from build123d import *

# Parameters (mm, degrees)
ESQUISSE1_W             = 23
ESQUISSE1_H             = 15.2
ESQUISSE1_R             = 1.5
BOSS_EXTRU_1_DEPTH      = 3
ESQUISSE2_W             = 23
ESQUISSE2_H             = 5
BOSS_EXTRU_2_DEPTH      = 10
ESQUISSE4_W             = 3
ESQUISSE4_H             = 31.2
BOSS_EXTRU_3_DEPTH      = 35
CONG_1_R                = 10
ESQUISSE7_W             = 10.405823793
ESQUISSE7_H             = 15
BOSS_EXTRU_4_DEPTH      = 3
ESQUISSE8_W             = 4
ESQUISSE8_H             = 15
BOSS_EXTRU_5_DEPTH      = 9.7
ESQUISSE9_W             = 26.005823793
ESQUISSE9_H             = 15
BOSS_EXTRU_6_DEPTH      = 5.52
ESQUISSE10_R            = 1.5
ENL_V_MAT_EXTRU_2_DEPTH = 5.52
ESQUISSE5_R             = 1.5
ENL_V_MAT_EXTRU_3_DEPTH = 10


with BuildPart() as part:
    # Esquisse1 → Boss.-Extru.1 (new body)
    with BuildSketch(Plane(origin=(0, 0, 0), x_dir=(0, 0, -1), z_dir=(1, 0, 0))):
        with Locations((11.5, -7.6)):
            Rectangle(ESQUISSE1_W, ESQUISSE1_H)
        with Locations((6.5, -5)):
            Circle(ESQUISSE1_R, mode=Mode.SUBTRACT)
        with Locations(Location((16.5, -5, 0), (0, 0, 180))):
            Circle(ESQUISSE1_R, mode=Mode.SUBTRACT)
    extrude(amount=BOSS_EXTRU_1_DEPTH)

    # Esquisse2 → Boss.-Extru.2 (add)
    with BuildSketch(Plane.ZY):
        with Locations((-11.5, -12.7)):
            Rectangle(ESQUISSE2_W, ESQUISSE2_H)
    boss_extru_2 = extrude(amount=BOSS_EXTRU_2_DEPTH)

    # Esquisse4 → Boss.-Extru.3 (add)
    with BuildSketch(Plane.XZ.offset(15.2)):
        with Locations((-8.5, -11.5)):
            Rectangle(ESQUISSE4_W, ESQUISSE4_H)
    boss_extru_3 = extrude(amount=BOSS_EXTRU_3_DEPTH)

    # Congé1
    cong_1_edges = [part.edges().sort_by_distance(p)[0] for p in [
        (-8.5, -50.2, -27.1),
        (-8.5, -50.2, 4.1),
    ]]
    fillet(cong_1_edges, radius=CONG_1_R)

    # Esquisse7 → Boss.-Extru.4 (add, through all)
    with BuildSketch(Plane(origin=(-7, 0, 0), x_dir=(0, 0, -1), z_dir=(1, 0, 0))):
        with Locations((-9.302911897, -27.2)):
            Rectangle(ESQUISSE7_W, ESQUISSE7_H)
    boss_extru_4 = extrude(amount=-BOSS_EXTRU_4_DEPTH)

    # Esquisse8 → Boss.-Extru.5 (add)
    with BuildSketch(Plane(origin=(-7, 0, 0), x_dir=(0, 0, -1), z_dir=(1, 0, 0))):
        with Locations((-12.505823793, -27.2)):
            Rectangle(ESQUISSE8_W, ESQUISSE8_H)
    boss_extru_5 = extrude(amount=BOSS_EXTRU_5_DEPTH)

    # Esquisse9 → Boss.-Extru.6 (add)
    with BuildSketch(Plane(origin=(2.7, 0, 0), x_dir=(0, 0, -1), z_dir=(1, 0, 0))):
        with Locations((-1.502911897, -27.2)):
            Rectangle(ESQUISSE9_W, ESQUISSE9_H)
    boss_extru_6 = extrude(amount=BOSS_EXTRU_6_DEPTH)

    # Symétrie1: Boss.-Extru.2, Boss.-Extru.3, Boss.-Extru.4, Boss.-Extru.5, Boss.-Extru.6 across plane
    add(boss_extru_2.mirror(Plane(origin=(8.22, -19.7, -11.5), x_dir=(1, 0, 0), z_dir=(0, 0, 1))))
    add(boss_extru_3.mirror(Plane(origin=(8.22, -19.7, -11.5), x_dir=(1, 0, 0), z_dir=(0, 0, 1))))
    add(boss_extru_4.mirror(Plane(origin=(8.22, -19.7, -11.5), x_dir=(1, 0, 0), z_dir=(0, 0, 1))))
    add(boss_extru_5.mirror(Plane(origin=(8.22, -19.7, -11.5), x_dir=(1, 0, 0), z_dir=(0, 0, 1))))
    add(boss_extru_6.mirror(Plane(origin=(8.22, -19.7, -11.5), x_dir=(1, 0, 0), z_dir=(0, 0, 1))))

    # Esquisse10 → Enlèv. mat.-Extru.2 (cut)
    with BuildSketch(Plane(origin=(8.22, 0, 0), x_dir=(0, 0, -1), z_dir=(1, 0, 0))):
        with BuildLine():
            ThreePointArc((3, -27.2), (1.5, -25.7), (0, -27.2))
            Line((0, -27.2), (3, -27.2))
        make_face()
        with BuildLine():
            Line((3, -27.2), (0, -27.2))
            ThreePointArc((0, -27.2), (1.5, -28.7), (3, -27.2))
        make_face()
        with BuildLine():
            Line((-4.4, -21.3), (-4.4, -27.2))
            Line((-4.4, -27.2), (0, -27.2))
            ThreePointArc((0, -27.2), (1.5, -25.7), (3, -27.2))
            Line((3, -27.2), (18.3, -27.2))
            Line((18.3, -27.2), (18.3, -21.3))
            Line((18.3, -21.3), (-4.4, -21.3))
        make_face()
        with BuildLine():
            Line((0, -27.2), (-4.4, -27.2))
            Line((-4.4, -27.2), (-4.4, -33.1))
            Line((-4.4, -33.1), (18.3, -33.1))
            Line((18.3, -33.1), (18.3, -27.2))
            Line((18.3, -27.2), (3, -27.2))
            ThreePointArc((3, -27.2), (1.5, -28.7), (0, -27.2))
        make_face()
        with Locations((-7.4, -27.2)):
            Circle(ESQUISSE10_R)
        with Locations((21.3, -27.2)):
            Circle(ESQUISSE10_R)
    extrude(amount=-ENL_V_MAT_EXTRU_2_DEPTH, mode=Mode.SUBTRACT)

    # Esquisse5 → Enlèv. mat.-Extru.3 (cut)
    with BuildSketch(Plane(origin=(-7, 0, 0), x_dir=(0, 0, -1), z_dir=(1, 0, 0))):
        with Locations((6.5, -45.2)):
            Circle(ESQUISSE5_R)
        with Locations((1.5, -27.2)):
            Circle(ESQUISSE5_R)
        with Locations((16.5, -45.2)):
            Circle(ESQUISSE5_R)
        with Locations((21.5, -27.2)):
            Circle(ESQUISSE5_R)
    extrude(amount=-ENL_V_MAT_EXTRU_3_DEPTH, mode=Mode.SUBTRACT)


solid = part.part
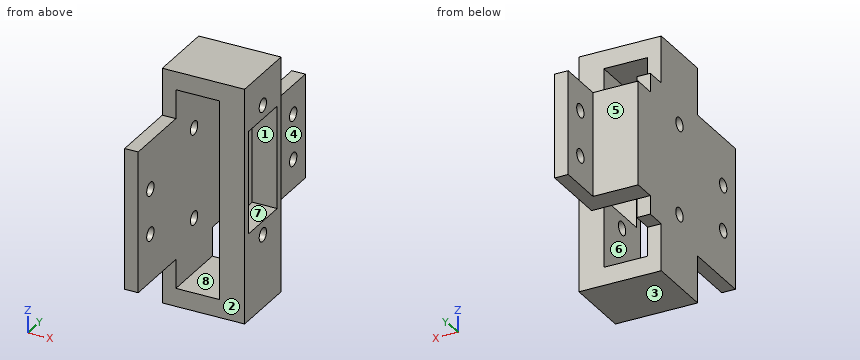
Read the model definition and answer for the solid it produces. Units are mm, in the model's axes. Face numbers are marked on the shaded views. A direction names the side the tool comes from. Round coordinates to 2 decimals unless told otherwise and drop trailing zeros. Order: outer loops, then holes, each group sorted by start corner. A loop starts at its lowest first (then second) coordinate and runs counter-clockwise, first axis right, second up.
1) The part is cut by section C-C on z = -1.5. Write down the section's boundary in (x, y).
2) The part is cut by section B-B on x = 1. Write down the section's boundary in (y, z).
3) For the marked faces 4, 5, 6, 7 and 8, determine the directions among +Z, -Z, +X, -X, +Y, -Y from which every point of the face is accessible in a straight line to the end or side of a thin tool.
4) The part is cut by section D-D on y = -5. Write down the section's boundary in (x, z), plus the area to 3 significant figures.
5) Flat-ended cylindrical pins translate along their axes: pin 1 (0.9 mm diameter, centred on x = -9, y = -43, fed in from -Z); pin 2 (8 mm diameter, centred on y = -4, z = -7, fed in from -X); pin 3 (4 mm diameter, centred on x = -4, z = -1.5, fed in from -Y). Find the tip coordinate at first contact, or state that the pin passes through.
6) The part is cut by section A-A on z = 7.4. Write down the section's boundary in (x, y), plus the area to 3 significant figures.
7) The mould has two halves that part along Z. Classify the marked faces 1, 2 and 3: released by +Z, released by -Z, zero draft, split by the parting line, or undercut.
8) Straight lines are drawn through the part: L1, parallel to Y at x = -8.2, z = -6.5; L2, parallel to Y at x = 7.1, z = 7.4; L3, parallel to Z at x = -0.75, y = -22. For each, find the intervals that lie inside material, in ascending order.
Resolved:
1. outline: (-10, -50.2) - (-7, -50.2) - (-7, -28.7) - (-10, -28.7) - close; (-10, -25.7) - (-7, -25.7) - (-7, -15.2) - (3, -15.2) - (3, 0) - (0, 0) - (0, -10.2) - (-10, -10.2) - close; (2.7, -34.7) - (8.22, -34.7) - (8.22, -33.1) - (2.7, -33.1) - close; (2.7, -21.3) - (8.22, -21.3) - (8.22, -19.7) - (2.7, -19.7) - close
2. outline: (-34.7, -37.51) - (-19.7, -37.51) - (-19.7, -33.51) - (-34.7, -33.51) - close; (-34.7, 10.51) - (-19.7, 10.51) - (-19.7, 14.51) - (-34.7, 14.51) - close; (-15.2, -23) - (0, -23) - (0, 0) - (-15.2, 0) - close; hole circle Ø3 at (-5, -16.5); hole circle Ø3 at (-5, -6.5)
3. face 4: +Z, -Z, +X, +Y
3. face 5: +Z, -Z, -X, +Y
3. face 6: -Y
3. face 7: +X
3. face 8: +Y, -Y
4. outline: (0, -23) - (3, -23) - (3, -18) - (0, -18) - close; (0, -15) - (3, -15) - (3, -8) - (0, -8) - close; (0, -5) - (3, -5) - (3, 0) - (0, 0) - close
4. area: 51.0 mm2
5. pin 1: stops at z = -27.1
5. pin 2: stops at x = 0
5. pin 3: stops at y = -15.2
6. outline: (-10, -34.7) - (-7, -34.7) - (-7, -19.7) - (-10, -19.7) - close; (2.7, -34.7) - (8.22, -34.7) - (8.22, -28.7) - (2.7, -28.7) - close; (2.7, -25.7) - (8.22, -25.7) - (8.22, -19.7) - (2.7, -19.7) - close
6. area: 111 mm2
7. face 1: undercut
7. face 2: zero draft
7. face 3: released by -Z
8. L1: y = -50.2 to -46.7, -43.7 to -10.2
8. L2: y = -34.7 to -28.7, -25.7 to -19.7
8. L3: z = -37.51 to -33.51, 10.51 to 14.51
